from build123d import *

# Parameters (mm, degrees)
CROQUIS1_R              = 1.6
SALIENTE_EXTRUIR3_DEPTH = 7.54
CROQUIS3_W              = 48.3
CROQUIS3_H              = 80
SALIENTE_EXTRUIR4_DEPTH = 15
CORTAR_EXTRUIR1_DEPTH   = 40.9
CROQUIS5_R              = 5
CORTAR_EXTRUIR2_DEPTH   = 54.9


with BuildPart() as part:
    # Croquis1 → Saliente-Extruir3 (new body)
    with BuildSketch(Plane.XY):
        Polygon((88.2, 0), (88.2, 37.6), (88.2, 58.8), (0, 58.8), (0, 37.6), (0, 0), (0, -21.2), (88.2, -21.2), align=None)
        with Locations((4.7, 34.4)):
            Circle(CROQUIS1_R, mode=Mode.SUBTRACT)
        with Locations((11.1, 34.4)):
            Circle(CROQUIS1_R, mode=Mode.SUBTRACT)
        with Locations((17.5, 34.4)):
            Circle(CROQUIS1_R, mode=Mode.SUBTRACT)
        with Locations((23.9, 34.4)):
            Circle(CROQUIS1_R, mode=Mode.SUBTRACT)
        with Locations((30.3, 34.4)):
            Circle(CROQUIS1_R, mode=Mode.SUBTRACT)
        with Locations((36.7, 34.4)):
            Circle(CROQUIS1_R, mode=Mode.SUBTRACT)
        with Locations((43.1, 34.4)):
            Circle(CROQUIS1_R, mode=Mode.SUBTRACT)
        with Locations((43.1, 3.2)):
            Circle(CROQUIS1_R, mode=Mode.SUBTRACT)
        with Locations((36.7, 3.2)):
            Circle(CROQUIS1_R, mode=Mode.SUBTRACT)
        with Locations((30.3, 3.2)):
            Circle(CROQUIS1_R, mode=Mode.SUBTRACT)
        with Locations((23.9, 3.2)):
            Circle(CROQUIS1_R, mode=Mode.SUBTRACT)
        with Locations((17.5, 3.2)):
            Circle(CROQUIS1_R, mode=Mode.SUBTRACT)
        with Locations((11.1, 3.2)):
            Circle(CROQUIS1_R, mode=Mode.SUBTRACT)
        with Locations((4.7, 3.2)):
            Circle(CROQUIS1_R, mode=Mode.SUBTRACT)
    extrude(amount=SALIENTE_EXTRUIR3_DEPTH)

    # Croquis3 → Saliente-Extruir4 (add)
    with BuildSketch(Plane(origin=(0, 0, 0), x_dir=(-1, 0, 0), z_dir=(0, 0, -1))):
        with Locations((-64.05, 18.8)):
            Rectangle(CROQUIS3_W, CROQUIS3_H)
    extrude(amount=SALIENTE_EXTRUIR4_DEPTH)

    # Croquis6 → Cortar-Extruir1 (cut)
    with BuildSketch(Plane.ZY):
        Polygon((0, 58.8), (2, 58.8), (2, -21.2), (0, -21.2), (-15, -21.2), (-15, 58.8), align=None)
    extrude(amount=-CORTAR_EXTRUIR1_DEPTH, mode=Mode.SUBTRACT)

    # Croquis5 → Cortar-Extruir2 (cut)
    with BuildSketch(Plane.ZY.offset(-39.9)):
        with Locations((-5, 42.36)):
            Circle(CROQUIS5_R)
        with Locations((-5, -4.76)):
            Circle(CROQUIS5_R)
    extrude(amount=-CORTAR_EXTRUIR2_DEPTH, mode=Mode.SUBTRACT)


solid = part.part
Geometry check sheet. Reference: the model listing, model coordinates, mm. A direction names the side the tool comes from. Give positions to 0.01 mm unless a question says otherwise; leave off trailing zeros. Write each loop counter-clockwise with the first axis right and the second up, starting at its lowest first coordinate (ties: lowest second). Pieces come first, ordered by that corner, then holes. Notation, with made-up numbers: (84, 55.25) - (120, 55.25) arc R11 ccw to (120, 61.25) - close; hole circle Ø7 at (41, -23.5). An arc over 180 degrees is marked (long way). Put each result on its own line as item: value.
1. Sectioned sample at C-C, the plane z = -5. Enter the section's corners in (x, y).
Ans:
outline: (40.9, -21.2) - (88.2, -21.2) - (88.2, -9.76) - (40.9, -9.76) - close; (40.9, 0.24) - (88.2, 0.24) - (88.2, 37.36) - (40.9, 37.36) - close; (40.9, 47.36) - (88.2, 47.36) - (88.2, 58.8) - (40.9, 58.8) - close
2. Sectioned sample at D-D, the plane y = 42.36. Enter the section's corners in (x, z).
Ans:
outline: (0, 2) - (40.9, 2) - (40.9, 0) - (88.2, 0) - (88.2, 7.54) - (0, 7.54) - close; (40.9, -15) - (88.2, -15) - (88.2, -10) - (40.9, -10) - close
3. Draft check along X on faces 4 (the cylindrical face through (5.44, 32.98, 4.73)), 5 (the flat face through (0, 19, 5)), 6 (the flat face through (88.2, 18, -4)). Enter one of: +X half, -X half, draft (parallel to the pull), parting line (faces both ways), or undercut.
Ans:
face 4: undercut
face 5: -X half
face 6: +X half
4. Sectioned sample at A-A, the plane y = 3.2. Give the number of separate pieces and of enclosed holes in the cut face, plus the area to 3 significant figures.
Ans:
separate pieces: 7
enclosed holes: 0
area: 1,160 mm²
5. Sectioned sample at B-B, the plane x = 11.1. Enter the section's corners in (y, z).
Ans:
outline: (-21.2, 2) - (1.6, 2) - (1.6, 7.54) - (-21.2, 7.54) - close; (4.8, 2) - (32.8, 2) - (32.8, 7.54) - (4.8, 7.54) - close; (36, 2) - (58.8, 2) - (58.8, 7.54) - (36, 7.54) - close
6. Go/stop test with flat-tipped pins: pin 1 (1.9 mm diameter, centred on x = 23.9, y = 34.4, fed in from +Z); pin 2 (10 mm diameter, centred on x = 30.5, z = -2, fed in from -Y); pin 3 (8 mm diameter, centred on y = 33, z = -7.5, fed in from -X); pin 4 (12 mm diameter, centred on x = 24.5, y = -10, fed in from -Z). Record where each tip stops, or that it passes through.
Ans:
pin 1: passes through
pin 2: stops at y = -21.2
pin 3: stops at x = 40.9
pin 4: stops at z = 2
7. Set-up check for faces 1 (the flat face through (20, 19, 2)), 2 (the cylindrical face through (43.84, 32.98, 3.72)), 3 (the cylindrical face through (6.18, 2.59, 4.73)): record each of +Z, -Z, +X, -X, +Y, -Y from which the full face is reachable in a straight line by a thin tool's end or side.
Ans:
face 1: -Z, -X, +Y, -Y
face 2: +Z
face 3: +Z, -Z
8. Thickness scan on line 1 (Y direction, x = 30.3, z = 3.3); line 2 (Y direction, x = 65, z = -5); line 3 (X direction, y = 18.5, z = -12.5). Record the ranges inside material, lowest first.
Ans:
line 1: y = -21.2 to 1.6, 4.8 to 32.8, 36 to 58.8
line 2: y = -21.2 to -9.76, 0.24 to 37.36, 47.36 to 58.8
line 3: x = 40.9 to 88.2
